Build history of the part. All positions in model axes, mm. Coordinates: 2 decimals unless noted, no trailing zeros. Loops run counter-clockwise (first coordinate to the right, second up) from the corner with the lowest first, then second, coordinate; pieces in that order, holes last.
(1) Slice it at B-B (x = -0.4). Give the cut face in (y, z).
(2) Wall check: L1, parallel to Z at x = 0.15, y = 11.5; L2, parallel to Z at x = -0.95, y = 22.5. Give the ranges that are in metal, low to high.
(3) Slice it at A-A (y = 17). Give the cut face in (x, z), and give its area (3 significant figures).
Solid Edge part; units mm, degrees
sketch "Sketch1" plane through (0, 0, 0) normal (0, -1, 0) x (1, 0, 0)
  line L0 (0.6, 31.75) -> (0.6, -31.75)
  line L1 (0.0064, -31.75) -> (0.6, -31.75)
  line L2 (-0.9936, -32.75) -> (0.0064, -31.75)
  line L3 (-1.5, -32.75) -> (-0.9936, -32.75)
  line L4 (-1.5, -32.75) -> (-1.5, 32.75)
  line L5 (-1.5, 32.75) -> (-0.9936, 32.75)
  line L6 (-0.9936, 32.75) -> (0.0064, 31.75)
  line L7 (0.0064, 31.75) -> (0.6, 31.75)
  dimension "D1" = 1.5
  dimension "D2" = 0.6
  dimension "D3" = 0.6
extrude "Protrusion1" add sketch "Sketch1" along normal mid plane 52
Response values:
1. outline: (-26, -32.16) - (26, -32.16) - (26, 32.16) - (-26, 32.16) - close
2. L1: z = -31.75 to 31.75
2. L2: z = -32.71 to 32.71
3. outline: (-1.5, -32.75) - (-0.99, -32.75) - (0.01, -31.75) - (0.6, -31.75) - (0.6, 31.75) - (0.01, 31.75) - (-0.99, 32.75) - (-1.5, 32.75) - close
3. area: 135 mm2
